Build history of the part. All positions in model axes, mm. A direction names the side the tool comes from. Round coordinates to 2 decimals unless told otherwise and drop trailing zeros. Loops run counter-clockwise (first coordinate to the right, second up) from the corner with the lowest first, then second, coordinate; pieces in that order, holes last. Notation, with made-up numbers: M 36.5,6 L 69.5,6 A28 cw 69.5,41 Z; hole C 64,85.25 d5. An arc over 180 degrees is marked long. Use one line per item in the form item = value. Start each with the question number.
```python
from build123d import *

# Parameters (mm, degrees)
ESQUISSE2_R        = 2
BOSS_EXTRU_1_DEPTH = 2.25
ESQUISSE3_R        = 1.5
BOSS_EXTRU_2_DEPTH = 2


with BuildPart() as part:
    # Esquisse2 → Boss.-Extru.1 (new body)
    with BuildSketch(Plane.XY):
        Circle(ESQUISSE2_R)
    boss_extru_1 = extrude(amount=BOSS_EXTRU_1_DEPTH)

    # Esquisse3 → Boss.-Extru.2 (add)
    with BuildSketch(Plane.XY.offset(2.25)):
        Circle(ESQUISSE3_R)
    boss_extru_2 = extrude(amount=BOSS_EXTRU_2_DEPTH)

    # Symétrie1: Boss.-Extru.1, Boss.-Extru.2 across plane
    add(boss_extru_1.mirror(Plane.XY))
    add(boss_extru_2.mirror(Plane.XY))


solid = part.part
```
Q1. Wall check: probe 1 along Z at (x, y) = (-1.2, -1.45); probe 2 along X at (y, z) = (-1.55, -2); probe 3 along Y at (x, z) = (-1.65, 0). Give the ranges that are in metal, low to high.
Q2. Tool access for faces 1 (the face through (0, -2, 0)), 2 (the face through (-1.5, 0.07, 3.24)), 3 (the face through (-1.5, 0.07, -3.24)): list every direction of +Z, -Z, +X, -X, +Y, -Y with a clear straight run to the whole face (end or side of a thin tool).
Q3. Drop flat-ended pins along their axis: P1, Ø1.5, axis at x = -0.5, z = -0.5, coming from the -Y side; P2, Ø2, axis at x = 1.5, z = 3.5, coming from the -Y side; P3, Ø1, axis at x = -1, z = 2.5, coming from the -Y side. Give the stop position or say it passes through.
Q4. Saw through at C-C (z = -0.5). Give the cut face in (x, y).
Q5. Saw through at A-A (x = 0). Give the cut face in (y, z).
Filled in:
q1.probe_1 = -2.25 to 2.25
q1.probe_2 = -1.26 to 1.26
q1.probe_3 = -1.13 to 1.13
q2.face_1 = +Z, -Z
q2.face_2 = +Z
q2.face_3 = -Z
q3.P1 = -2
q3.P2 = -1.41
q3.P3 = -1.92
q4.outline = C 0,0 d4
q5.outline = M -2,-2.25 L -1.5,-2.25 L -1.5,-4.25 L 1.5,-4.25 L 1.5,-2.25 L 2,-2.25 L 2,2.25 L 1.5,2.25 L 1.5,4.25 L -1.5,4.25 L -1.5,2.25 L -2,2.25 Z
